Read the model definition and answer for the solid it produces. Units are mm, in the model's axes. A direction names the side the tool comes from. Give positions to 0.01 mm unless a question says otherwise; leave off trailing zeros. Order: outer loops, then holes, each group sorted by start corner. A loop starts at its lowest first (then second) coordinate and runs counter-clockwise, first axis right, second up. Notation, with made-up numbers: M -3.5,61.5 L 5.5,61.5 A27 cw 5.5,79.5 Z; hole C 20.5,-8.5 d5. An arc over 180 degrees is marked long. One line per item, written item: value. Start each with the question number.
from build123d import *

# Parameters (mm, degrees)
ESQUISSE1_W        = 30
ESQUISSE1_H        = 10
BOSS_EXTRU_1_DEPTH = 35
ESQUISSE3_R        = 1
BOSS_EXTRU_2_DEPTH = 15
ESQUISSE4_W        = 35
ESQUISSE4_H        = 75
BOSS_EXTRU_3_DEPTH = 14


with BuildPart() as part:
    # Esquisse1 → Boss.-Extru.1 (new body)
    with BuildSketch(Plane(origin=(0, 0, 0), x_dir=(0, 0, -1), z_dir=(1, 0, 0))):
        with Locations((23.668323467, -1.396462247)):
            Rectangle(ESQUISSE1_W, ESQUISSE1_H)
    extrude(amount=BOSS_EXTRU_1_DEPTH)

    # Esquisse3 → Boss.-Extru.2 (add)
    with BuildSketch(Plane(origin=(35, 0, 0), x_dir=(0, 0, -1), z_dir=(1, 0, 0))):
        with Locations((13.450280626, -1.396462247)):
            Circle(ESQUISSE3_R)
    extrude(amount=BOSS_EXTRU_2_DEPTH)

    # Esquisse4 → Boss.-Extru.3 (add)
    with BuildSketch(Plane(origin=(35, 0, 0), x_dir=(0, 0, -1), z_dir=(1, 0, 0))):
        with Locations((23.668323467, -33.896462247)):
            Rectangle(ESQUISSE4_W, ESQUISSE4_H)
    extrude(amount=-BOSS_EXTRU_3_DEPTH)


solid = part.part
Q1. Consider probe 1 along X at (y, z) = (-63, -9.5); probe 2 along Y at (x, z) = (7, -37); probe 3 along Z at (x, y) = (18, 0). Determine where each line is inside the solid, lowest interval first.
Q2. A tool of negligible diameter and unlimited length cuts with its end or side. For faces 1 (the cylindrical face through (42.395, -0.553, -13.988)), 2 (the flat face through (10, -1, -8.668)), 3 (the flat face through (10, -1, -38.668)), 4 (the flat face through (10, -6.396, -23)), from which of +Z, -Z, +X, -X, +Y, -Y can it reach the whole face along a straight path? Write none if from no direction.
Q3. Find section C-C, the plane x = 14. Give the vertices of the cut face in (y, z), then the cut area to 3 significant figures.
Q4. Find section B-B, the plane y = -62.5. Give the vertices of the cut face in (x, z), then the cut area to 3 significant figures.
Q5. Find section A-A, the plane z = -27. Give the vertices of the cut face in (x, y).
Q6. Each of these flat-tipped pins is pushed along its axis until it touches: pin 1 (10.5 mm diameter, centred on x = 13, z = -28.5, fed in from -Y); pin 2 (5 mm diameter, centred on x = 13.5, y = -1.5, fed in from -Z); pin 3 (1.5 mm diameter, centred on y = -52.5, z = -12.5, fed in from +X). Where does it stop, or does it pass through?
Evaluation:
1. probe 1: 21 to 35
1. probe 2: -6.4 to 3.6
1. probe 3: -38.67 to -8.67
2. face 1: +X
2. face 2: +Z, -X, +Y, -Y
2. face 3: -Z, -X, +Y, -Y
2. face 4: +Z, -Z, -X, -Y
3. outline: M -6.4,-38.67 L 3.6,-38.67 L 3.6,-8.67 L -6.4,-8.67 Z
3. area: 300 mm2
4. outline: M 21,-41.17 L 35,-41.17 L 35,-6.17 L 21,-6.17 Z
4. area: 490 mm2
5. outline: M 0,-6.4 L 21,-6.4 L 21,-71.4 L 35,-71.4 L 35,3.6 L 0,3.6 Z
6. pin 1: y = -6.4
6. pin 2: z = -38.67
6. pin 3: x = 35
